```python
from build123d import *

# Parameters (mm, degrees)
F0_R     = 2.25
F1_DEPTH = 10
F2_R     = 1


with BuildPart() as f1:
    # F0 (on Top) → F1 (new body)
    with BuildSketch(Plane.XY):
        with BuildLine():
            ThreePointArc((9.5009885105, -8.1228823285), (11.7263028355, -4.3294135641), (12.5, 0))
            ThreePointArc((12.5, 0), (12.3770625391, 1.7488061363), (12.0106683356, 3.4632132668))
            ThreePointArc((12.0106683356, 3.4632132668), (8.2330297979, 9.4057014808), (1.8427561446, 12.3634238701))
            ThreePointArc((1.8427561446, 12.3634238701), (-4.5491075048, 11.6428356044), (-9.7363625852, 7.8392119253))
            Line((-9.7363625852, 7.8392119253), (-7.8092353717, 6.240187919))
            ThreePointArc((-7.8092353717, 6.240187919), (3.3061601135, 9.4336317322), (9.9962043974, 0))
            ThreePointArc((9.9962043974, 0), (9.3710716558, -3.4795284703), (7.573861297, -6.5238583222))
            Line((7.573861297, -6.5238583222), (9.5009885105, -8.1228823285))
        make_face()
        with BuildLine():
            ThreePointArc((1.8427561446, 12.3634238701), (8.2330297979, 9.4057014808), (12.0106683356, 3.4632132668))
            Line((12.0106683356, 3.4632132668), (88.4712676923, 96.0025354569))
            Line((88.4712676923, 96.0025354569), (80.951972171, 102.5949701258))
            Line((80.951972171, 102.5949701258), (1.8427561446, 12.3634238701))
        make_face()
        with Locations((81.4098492265, 95.7288071513)):
            Circle(F0_R, mode=Mode.SUBTRACT)
    extrude(amount=F1_DEPTH)

    # F2
    f2_edges = [f1.edges().sort_by_distance(p)[0] for p in [
        (41.397364, 57.479197, 10),
        (12.216679, -2.646271, 10),
        (50.240968, 49.732874, 10),
        (-4.549108, 11.642836, 10),
        (12.216679, -2.646271, 0),
        (-4.549108, 11.642836, 0),
        (50.240968, 49.732874, 0),
        (41.397364, 57.479197, 0),
        (79.159849, 95.728807, 0),
        (84.71162, 99.298753, 0),
        (79.159849, 95.728807, 10),
        (88.471268, 96.002535, 5),
        (80.951972, 102.59497, 5),
        (84.71162, 99.298753, 10),
    ]]
    fillet(f2_edges, radius=F2_R)


solid = f1.part
```
Can you work these out from the model? Positions are in its coordinate system, mm. Round coordinates to 2 decimals unless told otherwise and drop trailing zeros. Order: outer loops, then holes, each group sorted by start corner. A loop starts at its lowest first (then second) coordinate and runs counter-clockwise, first axis right, second up.
(1) If I drill on L1, parallel to Y at x = 64, z = 8; L2, parallel to X at y = 63, z = 2.75; L3, parallel to Y at x = 26.5, z = 6, over which ranges is the centre line in solid material (lowest first)?
Results are:
L1: y = 66.39 to 83.26
L2: x = 46.24 to 61.2
L3: y = 21 to 40.49
(2) If we section it at A-A (z = 3.75): Please give me the cut outline in (x, y).
Results are:
outline: (-9.74, 7.84) - (-7.81, 6.24) arc R10 cw (long way) to (7.57, -6.52) - (9.5, -8.12) arc R12.5 ccw to (12.01, 3.46) - (87.85, 95.25) arc R1 ccw to (87.74, 96.64) - (81.7, 101.94) arc R1 ccw to (80.29, 101.84) - (1.84, 12.36) arc R12.5 ccw to start; hole circle Ø4.5 at (81.41, 95.73)
(3) We'd pull the mould along X, two halves only. Please class faces 1 (the face through (39, 47, 10)), 2 (the face through (83.5, 94.9, 4.9)), 3 (the face through (50.073, 49.977, 0.301)): +X half, -X half, draft (parallel to the pull), parting line (faces both ways), or undercut.
Results are:
face 1: draft
face 2: undercut
face 3: +X half
(4) I'm going to push flat-ended pins straight in: pin 1 (1.5 mm diameter, centred on x = 16.5, z = 6, fed in from -Y); pin 2 (2 mm diameter, centred on x = 57.5, z = 5.5, fed in from +Y); pin 3 (2 mm diameter, centred on x = 17.5, z = 6.5, fed in from -Y). Where does each tip first touch, or does it pass through?
Results are:
pin 1: stops at y = 7.99
pin 2: stops at y = 76.99
pin 3: stops at y = 8.9
